The model under review builds one solid part; all positions refer to its coordinate system, in mm. A direction names the side the tool comes from. Give positions to 0.01 mm unless a question says otherwise; leave off trailing zeros. Order: outer loops, then holes, each group sorted by start corner. A loop starts at its lowest first (then second) coordinate and runs counter-clockwise, first axis right, second up.
```python
from build123d import *

# Parameters (mm, degrees)
F0_R      = 7.84357
F0_R_2    = 7.775719
F1_DEPTH  = 5.67
F2_W      = 17.690338
F2_H      = 15.67
F3_DEPTH  = 5.67
F4_R      = 1.425
F5_DEPTH  = 10.38
F6_R      = 1.425
F7_DEPTH  = 10.38
F9_R      = 2.465
F10_DEPTH = 2.425
F11_W     = 13.306394
F11_H     = 11.622041
F12_DEPTH = 3
F13_R     = 2.75
F13_R_2   = 1.75
F14_DEPTH = 2


with BuildPart() as f1:
    # F0 (on Front) → F1 (new body)
    with BuildSketch(Plane.XZ):
        with Locations((-31.018244, 13.502214)):
            Circle(F0_R)
        with Locations((27.656266, 13.502214)):
            Circle(F0_R_2)
        with Locations((-31.018244, -35.786617)):
            Circle(F0_R_2)
        with Locations((27.656266, -35.786617)):
            Circle(F0_R_2)
    extrude(amount=F1_DEPTH)


with BuildPart() as f3:
    # F2 (on Front) → F3 (new body)
    with BuildSketch(Plane.XZ):
        with Locations((-76.058906, 37.108815)):
            Rectangle(F2_W, F2_H)
    extrude(amount=F3_DEPTH)

    # F4 (on face) → F5 (join)
    with BuildSketch(Plane(origin=(-84.904075, 0, 0), x_dir=(0, -1, 0), z_dir=(-1, 0, 0))):
        with Locations((2.974371, 37.108815)):
            Circle(F4_R)
    extrude(amount=F5_DEPTH)

    # F6 (on face) → F7 (join)
    with BuildSketch(Plane.YZ.offset(-67.213737)):
        with Locations((-3.072243, 37.108815)):
            Circle(F6_R)
    extrude(amount=F7_DEPTH)

    # F9 (on face) → F10 (join)
    with BuildSketch(Plane.XZ.offset(5.67)):
        with Locations((-79.964688, 41.62437)):
            Circle(F9_R)
        with Locations((-71.483449, 41.62437)):
            Circle(F9_R)
        with Locations((-79.964688, 34.203287)):
            Circle(F9_R)
        with Locations((-71.483449, 34.600842)):
            Circle(F9_R)
    extrude(amount=F10_DEPTH)

    # F11 (on face) → F12 (cut)
    with BuildSketch(Plane(origin=(0, 0, 0), x_dir=(-1, 0, 0), z_dir=(0, 1, 0))):
        with Locations((76.318003, 37.002533)):
            Rectangle(F11_W, F11_H)
    extrude(amount=-F12_DEPTH, mode=Mode.SUBTRACT)

    # F13 (on face) → F14 (join)
    with BuildSketch(Plane(origin=(0, -3, 0), x_dir=(-1, 0, 0), z_dir=(0, 1, 0))):
        with Locations((76.065354, 37.592057)):
            Circle(F13_R)
        with Locations((76.065354, 37.592057)):
            Circle(F13_R_2, mode=Mode.SUBTRACT)
    extrude(amount=F14_DEPTH)


solid = f3.part
```
Item 1: For faces 4 (the flat face through (-76, -3, 29.274)), 5 (the flat face through (-76, -1, 42.814)), 6 (the cylindrical face through (-81.78, -6.87, 35.87)), 7 (the cylindrical face through (-90.02, -2.79, 38.52)), list the 3-axis set-ups (+Z, -Z, +X, -X, +Y, -Y) from which the entire face can be reached by the end or side of a thin tool; tool diameter is ignored.
Values found:
face 4: -Z, +X, -X, +Y, -Y
face 5: +Y
face 6: -Y
face 7: -X
Item 2: Take a section at D-D (y = -6.75). Give the boundary of the cut face in (x, z) (3 decimals).
Values found:
outline: circle Ø4.93 at (-79.965, 34.203); circle Ø4.93 at (-79.965, 41.624); circle Ø4.93 at (-71.483, 34.601); circle Ø4.93 at (-71.483, 41.624)
Item 3: Draft analysis for pull direction X (two halves, no side actions). For faces 1 (the flat face through (-76, -3, 44.944)), 2 (the flat face through (-84.904, -3, 35)), 3 (the cylindrical face through (-73.3, -6.87, 36.27)), state which applies: released by +X, released by -X, zero draft, split by the parting line, or undercut.
Values found:
face 1: zero draft
face 2: released by -X
face 3: undercut
Item 4: Clearance check with flat-ended pins moving along their axes: pin 1 Ø8 at (x, z) = (-67.5, 43) entering from +Y; pin 2 Ø4 at (x, z) = (-77, 37.5) entering from +Y; pin 3 Ø3 at (y, z) = (-1.5, 40) entering from +X; pin 4 Ø2 at (x, z) = (-76.07, 37.59) entering from +Y. State where each tip first meets the part, or that it passes through.
Values found:
pin 1: stops at y = 0
pin 2: stops at y = -1
pin 3: stops at x = -67.21
pin 4: stops at y = -3
Item 5: For line 1 (X direction, y = -2.75, z = 31.5); line 2 (Z direction, x = -79.5, y = -1); line 3 (Y direction, x = -72, z = 31), list the stretches that pass through material, from the lowest coordinate up.
Values found:
line 1: x = -84.9 to -82.97, -69.66 to -67.21
line 2: z = 29.27 to 31.19, 42.81 to 44.94
line 3: y = -5.67 to 0
Item 6: Take a section at C-C (x = -77). Give the boundary of the cut face in (y, z).
Values found:
outline: (-5.67, 29.27) - (0, 29.27) - (0, 31.19) - (-3, 31.19) - (-3, 35.01) - (-1, 35.01) - (-1, 36.11) - (-3, 36.11) - (-3, 39.07) - (-1, 39.07) - (-1, 40.18) - (-3, 40.18) - (-3, 42.81) - (0, 42.81) - (0, 44.94) - (-5.67, 44.94) - close
Item 7: Take a section at B-B (z = 41.25). Give the boundary of the cut face in (x, y) (3 decimals), and give its area (3 significant figures).
Values found:
outline: (-84.904, -5.67) - (-82.401, -5.67) - (-82.401, -8.095) - (-77.528, -8.095) - (-77.528, -5.67) - (-73.92, -5.67) - (-73.92, -8.095) - (-69.047, -8.095) - (-69.047, -5.67) - (-67.214, -5.67) - (-67.214, 0) - (-69.665, 0) - (-69.665, -3) - (-82.971, -3) - (-82.971, 0) - (-84.904, 0) - close
area: 84.0 mm2
Item 8: Take a section at A-A (y = -2). Give the boundary of the cut face in (x, z), and give its area (3 significant figures).
Values found:
outline: (-95.28, 36.07) - (-84.9, 36.07) - (-84.9, 29.27) - (-67.21, 29.27) - (-67.21, 36.17) - (-56.83, 36.17) - (-56.83, 38.05) - (-67.21, 38.05) - (-67.21, 44.94) - (-84.9, 44.94) - (-84.9, 38.15) - (-95.28, 38.15) - close; circle Ø5.5 at (-76.07, 37.59); hole (-82.97, 31.19) - (-69.66, 31.19) - (-69.66, 42.81) - (-82.97, 42.81) - close; hole circle Ø3.5 at (-76.07, 37.59)
area: 178 mm2
